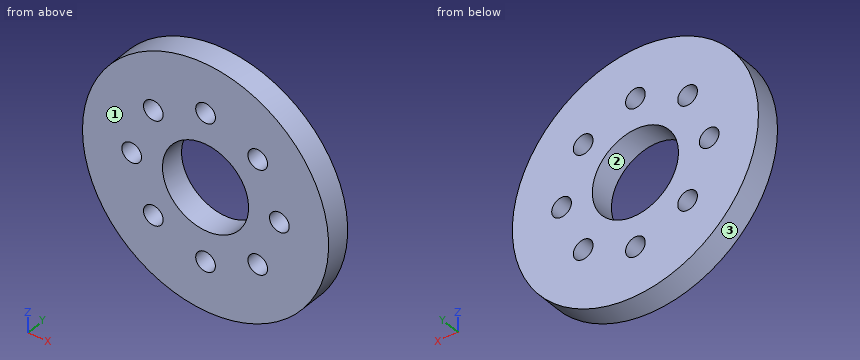
Autodesk Inventor part; units mm, degrees
ref_plane "YZ Plane" through (0, 0, 0) normal (1, 0, 0) x (0, 1, 0)
ref_plane "XZ Plane" through (0, 0, 0) normal (0, 1, 0) x (-1, 0, 0)
ref_plane "XY Plane" through (0, 0, 0) normal (0, 0, 1) x (1, 0, 0)
sketch "Sketch1" plane through (0, 0, 0) normal (0, 1, 0) x (-1, 0, 0)
  circle A0 centre (0, 0) radius 50
  dimension "d1" = 100
extrude "Extrusion1" add sketch "Sketch1" along normal blind 10
sketch "Sketch2" plane through (0, 10, 0) normal (0, 1, 0) x (1, 0, 0)
  circle A0 centre (0, 0) radius 16
  dimension "d4" = 32
hole "Hole1" at (0, 10, 0) direction (0, -1, 0) diameter 35 end through all
sketch "Sketch3" plane through (0, 10, 0) normal (0, 1, 0) x (1, 0, 0)
  circle A0 centre (0, 30) radius 4
  circle A1 centre (-21.2132, 21.2132) radius 4
  circle A2 centre (-30, 0) radius 4
  circle A3 centre (-21.2132, -21.2132) radius 4
  circle A4 centre (0, -30) radius 4
  circle A5 centre (21.2132, -21.2132) radius 4
  circle A6 centre (30, 0) radius 4
  circle A7 centre (21.2132, 21.2132) radius 4
  point P0 (0, 0)
  point P1 (0, 0)
  dimension "d12" = 8
  dimension "d13" = 30
  dimension "d16" = 360
hole "Hole2" at (-21.2132, 10, 21.2132) at (-30, 10, 0) at (-21.2132, 10, -21.2132) at (0, 10, -30) at (21.2132, 10, -21.2132) at (30, 10, 0) at (21.2132, 10, 21.2132) at (0, 10, 30) direction (0, -1, 0) diameter 8 end through all
sketch "Sketch4" plane through (0, 10, 0) normal (0, 1, 0) x (1, 0, 0)
  point P0 (0, 0)
properties part number "Orifice Plate" material "Aluminum 6061"
The listing builds one solid part. Answer for the finished solid, in the listing's coordinates (mm). Face numbers are marked on the shaded views. Round coordinates to 2 decimals unless told otherwise and drop trailing zeros. Write each loop counter-clockwise with the first axis right and the second up, starting at its lowest first coordinate (ties: lowest second). Pieces come first, ordered by that corner, then holes. Notation, with made-up numbers: (84.5, -29.5) -> (117.5, -29.5) arc R20 ccw to (117.5, -1.5) -> close; hole circle Ø9 at (73.25, 37). An arc over 180 degrees is marked (long way). Write item = value, one per line.
1) Section A-A on z = -30 is taken. Write down the section's boundary in (x, y), plus the area to 3 significant figures.
Check values:
outline = (-40, 0) -> (-4, 0) -> (-4, 10) -> (-40, 10) -> close; (4, 0) -> (40, 0) -> (40, 10) -> (4, 10) -> close
area = 720 mm²
2) Section D-D on y = 4.5 is taken. Give the number of separate pieces and of enclosed holes in the cut face, plus the area to 3 significant figures.
Check values:
separate_pieces = 1
enclosed_holes = 9
area = 6,490 mm²
3) For a pull along Z with two mould halves and no side action, classify the marked faces 1, 2 and 3 as released by +Z, released by -Z, zero draft, split by the parting line, or undercut.
Check values:
face_1 = zero draft
face_2 = undercut
face_3 = split by the parting line
4) Straight lines are drawn through the part: line 1 along Z through (x, y) = (0, 1.5); line 2 along X through (y, z) = (8, -2); line 3 along X through (y, z) = (4.25, 24). For each, find the intervals that lie inside material, in ascending order. Write a range as [from, to].
Check values:
line_1 = [-50, -34], [-26, -17.5], [17.5, 26], [34, 50]
line_2 = [-49.96, -33.46], [-26.54, -17.39], [17.39, 26.54], [33.46, 49.96]
line_3 = [-43.86, -24.08], [-18.34, 18.34], [24.08, 43.86]
5) Given pin 1 (7 mm diameter, centred on x = 21.21, z = 21.21, fed in from -Y); pin 2 (5 mm diameter, centred on x = 23, y = 3, fed in from -Z); pin 3 (3 mm diameter, centred on y = 2.5, z = -18, fed in from -X); pin 4 (6 mm diameter, centred on x = 30.5, y = 1.5, fed in from +Z), each flat-ended and moving along its own axis, determine where each tip first touches the part or whether it passes through.
Check values:
pin_1 = through
pin_2 = -45.6
pin_3 = -47.2
pin_4 = 41.76
6) Section C-C on x = 0 is taken. Write down the section's boundary in (y, z).
Check values:
outline = (0, -50) -> (10, -50) -> (10, -34) -> (0, -34) -> close; (0, -26) -> (10, -26) -> (10, -17.5) -> (0, -17.5) -> close; (0, 17.5) -> (10, 17.5) -> (10, 26) -> (0, 26) -> close; (0, 34) -> (10, 34) -> (10, 50) -> (0, 50) -> close
7) Section B-B on x = 30 is taken. Write down the section's boundary in (y, z).
Check values:
outline = (0, -40) -> (10, -40) -> (10, -4) -> (0, -4) -> close; (0, 4) -> (10, 4) -> (10, 40) -> (0, 40) -> close
